Source: CAD feature listing. Evaluate the final solid. Frame: model axes, mm. A direction names the side the tool comes from. Give positions to 0.01 mm unless a question says otherwise; leave off trailing zeros. Write each loop counter-clockwise with the first axis right and the second up, starting at its lowest first coordinate (ties: lowest second). Pieces come first, ordered by that corner, then holes. Notation, with made-up numbers: (-26, 39.5) -> (24, 39.5) arc R29 cw to (24, 72.5) -> close; hole circle Ø3 at (26.25, -32.75). An arc over 180 degrees is marked (long way). Answer as a JSON object with one key per item and string values. Group by question number.
Item 1: First-contact query: pin 1 Ø10 at (x, z) = (112.5, -30.5) entering from -Y. Flat tip, straight axial feed; report the tip coordinate or a pass-through.
Item 2: Section query A-A on z = -27.5. Return the cut outline in (x, y) (3 decimals).
Item 3: Section query C-C on y = 2. Return the cut outline in (x, z), plus the area to 3 significant figures.
Item 4: Pull-direction query (Z, two-part tool) for faces 1 (the face through (140, 2, -49)), 2 (the face through (73, 2, -30)), 3 (the face through (11, 2, 0)), 4 (the face through (114, 2, -30)); classes: pulls with the +Z half, pulls with the -Z half, needs draft (parallel to the pull), parting line crosses it, or undercut.
Item 5: Ray query, probe 1 along Z at (x, y) = (96, 2.35); probe 2 along X at (y, z) = (1.45, -12); probe 3 along X at (y, z) = (1.2, -11.5). Return the intervals inside material, ascending. Write a range as from..to.
Item 6: Section query D-D on x = 55.5. Return the cut outline in (y, z) (3 decimals).
Item 7: Access query for faces 5 (the face through (93, 2, -40.51)), 6 (the face through (69, 0, -51)). Directions: +Z, -Z, +X, -X, +Y, -Y. A direction counts if a zero-diameter tool reaches every point of the face in a straight line with its end or side. Return the directions, or none.
Item 8: Section query B-B on x = 110. Return the cut outline in (y, z) (3 decimals).
from build123d import *

# Parameters (mm, degrees)
SKETCH1_W           = 140
SKETCH1_H           = 100
BOSS_EXTRUDE1_DEPTH = 3.175
SKETCH2_W           = 41
SKETCH2_H           = 20
CUT_EXTRUDE1_DEPTH  = 10
SKETCH3_R           = 30
CUT_EXTRUDE2_DEPTH  = 10


with BuildPart() as part:
    # Sketch1 → Boss-Extrude1 (new body)
    with BuildSketch(Plane(origin=(0, 0, 0), x_dir=(1, 0, 0), z_dir=(0, 1, 0))):
        with Locations((70, 50)):
            Rectangle(SKETCH1_W, SKETCH1_H)
    extrude(amount=BOSS_EXTRUDE1_DEPTH)

    # Sketch2 → Cut-Extrude1 (cut)
    with BuildSketch(Plane(origin=(0, 3.175, 0), x_dir=(1, 0, 0), z_dir=(0, 1, 0))):
        with Locations((93.5, 30.51)):
            Rectangle(SKETCH2_W, SKETCH2_H)
    extrude(amount=-CUT_EXTRUDE1_DEPTH, mode=Mode.SUBTRACT)

    # Sketch3 → Cut-Extrude2 (cut)
    with BuildSketch(Plane(origin=(0, 3.175, 0), x_dir=(1, 0, 0), z_dir=(0, 1, 0))):
        with Locations((50, -10)):
            Circle(SKETCH3_R)
    extrude(amount=-CUT_EXTRUDE2_DEPTH, mode=Mode.SUBTRACT)


solid = part.part
Worked answers:
{
 "1": {"pin 1": "y = 0"},
 "2": {"outline": "(0, 0) -> (73, 0) -> (73, 3.175) -> (0, 3.175) -> close; (114, 0) -> (140, 0) -> (140, 3.175) -> (114, 3.175) -> close"},
 "3": {"outline": "(0, -100) -> (140, -100) -> (140, 0) -> (78.28, 0) arc R30 cw to (21.72, 0) -> (0, 0) -> close; hole (73, -40.51) -> (114, -40.51) -> (114, -20.51) -> (73, -20.51) -> close", "area": "12,400 mm^2"},
 "4": {"face 1": "needs draft", "face 2": "undercut", "face 3": "pulls with the +Z half", "face 4": "undercut"},
 "5": {"probe 1": "-100..-40.51, -20.51..0", "probe 2": "0..29.6, 70.4..140", "probe 3": "0..29.08, 70.92..140"},
 "6": {"outline": "(0, -100) -> (3.175, -100) -> (3.175, -19.492) -> (0, -19.492) -> close"},
 "7": {"face 5": "+Y, -Y", "face 6": "+Z, -Z, +X, -X, -Y"},
 "8": {"outline": "(0, -100) -> (3.175, -100) -> (3.175, -40.51) -> (0, -40.51) -> close; (0, -20.51) -> (3.175, -20.51) -> (3.175, 0) -> (0, 0) -> close"}
}
